from build123d import *

# Parameters (mm, degrees)
SKETCH1_R           = 1.5
BOSS_EXTRUDE1_DEPTH = 2
SKETCH2_R           = 1.5
BOSS_EXTRUDE2_DEPTH = 5
CUT_EXTRUDE1_DEPTH  = 2
SKETCH5_W           = 3
SKETCH5_H           = 1
CUT_EXTRUDE2_DEPTH  = 22


with BuildPart() as part:
    # Sketch1 → Boss-Extrude1 (new body)
    with BuildSketch(Plane.XY):
        Polygon((-8, 3.5), (-6, 5.5), (6, 5.5), (8, 3.5), (8, -3.5), (6, -5.5), (-6, -5.5), (-8, -3.5), align=None)
        with Locations((-2.5, 0)):
            Circle(SKETCH1_R, mode=Mode.SUBTRACT)
        with Locations((2.5, 0)):
            Circle(SKETCH1_R, mode=Mode.SUBTRACT)
    extrude(amount=BOSS_EXTRUDE1_DEPTH)

    # Sketch2 → Boss-Extrude2 (add)
    with BuildSketch(Plane.XY.offset(2)):
        with BuildLine():
            Line((-2.5, 4.5), (2.5, 4.5))
            ThreePointArc((2.5, 4.5), (7, 0), (2.5, -4.5))
            Line((2.5, -4.5), (-2.5, -4.5))
            ThreePointArc((-2.5, -4.5), (-7, 0), (-2.5, 4.5))
        make_face()
        with Locations((-2.5, 0)):
            Circle(SKETCH2_R, mode=Mode.SUBTRACT)
        with Locations((2.5, 0)):
            Circle(SKETCH2_R, mode=Mode.SUBTRACT)
    extrude(amount=BOSS_EXTRUDE2_DEPTH)

    # Sketch4 → Cut-Extrude1 (cut)
    with BuildSketch(Plane.XY.offset(7)):
        with BuildLine():
            Line((-2.5, -2.5), (2.5, -2.5))
            ThreePointArc((2.5, -2.5), (3.618033989, -2.236067977), (4.5, -1.5))
            Line((4.5, -1.5), (7.291771179, -1.5))
            Line((7.291771179, -1.5), (6.980260776, 3.5))
            Line((6.980260776, 3.5), (4.540127242, 3.5))
            Line((4.540127242, 3.5), (-4.895055756, 3.5))
            Line((-4.895055756, 3.5), (-6.610543574, 3.5))
            Line((-6.610543574, 3.5), (-7.482128219, -1.5))
            Line((-7.482128219, -1.5), (-4.5, -1.5))
            ThreePointArc((-4.5, -1.5), (-3.618033989, -2.236067977), (-2.5, -2.5))
        make_face()
    extrude(amount=-CUT_EXTRUDE1_DEPTH, mode=Mode.SUBTRACT)

    # Sketch5 → Cut-Extrude2 (cut)
    with BuildSketch(Plane.ZY.offset(8)):
        with Locations((5.5, 4)):
            Rectangle(SKETCH5_W, SKETCH5_H)
    extrude(amount=-CUT_EXTRUDE2_DEPTH, mode=Mode.SUBTRACT)


solid = part.part
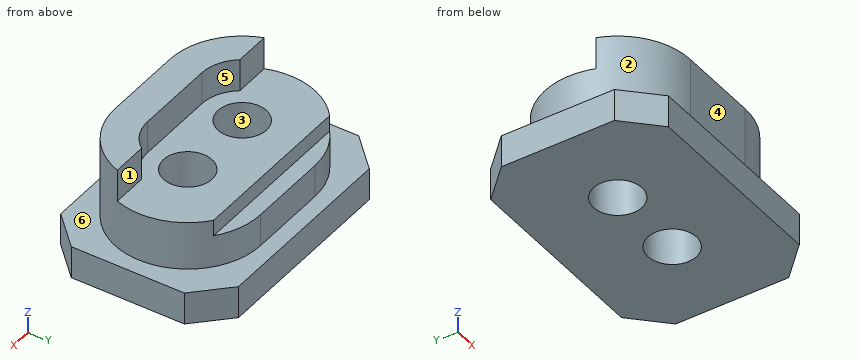
Here's how the part is built. I have some questions about the finished solid (model axes, mm). Face numbers are marked on the shaded views. A direction names the side the tool comes from. Give positions to 0.01 mm unless a question says otherwise; leave off trailing zeros. Loops run counter-clockwise (first coordinate to the right, second up) from the corner with the lowest first, then second, coordinate; pieces in that order, holes last. Notation, with made-up numbers: (16.5, 63.25) -> (44.5, 63.25) arc R12 cw to (44.5, 72.25) -> close; hole circle Ø2 at (-37, 7.5). An arc over 180 degrees is marked (long way). Answer as a JSON object with one key per item and string values. Group by question number.
Item 1: Imagine slicing it at B-B on y = 0. Write out the boundary of the cut face in (x, z).
Item 2: Thinking about a two-plate mould opening in X: for the marked faces 1, 2 and 3, which applies, pulls with the +X half, pulls with the -X half, needs draft (parallel to the pull), parting line crosses it, or undercut?
Item 3: Imagine slicing it at A-A on z = 0.5. Write out the boundary of the cut face in (x, y).
Item 4: On a 3-axis mill with a long thin cutter (end or side, diameter ignored), from which of +Z, -Z, +X, -X, +Y, -Y can I reach the whole of each face in a straight line? I mean the marked faces 4, 5 and 6. Say none if no direction works.
Item 5: Imagine slicing it at D-D on z = 5.25. Write out the boundary of the cut face in (x, y), then the cut area to 3 significant figures.
Item 6: Imagine slicing it at C-C on x = 2. Write out the boundary of the cut face in (y, z).
Item 7: Will these pins go through, and if not, where does the flat tip stop? pin 1 (0.8 mm diameter, centred on x = 0, z = 4.5, fed in from +Y); pin 2 (1.6 mm diameter, centred on x = -6, z = 6, fed in from +Y); pin 3 (0.6 mm diameter, centred on x = -1, z = 3, fed in from +Y); pin 4 (1.8 mm diameter, centred on x = 2.5, y = 0, fed in from +Z).
Item 8: I need wall thicknesses on L1, parallel to X at y = 0, z = 2.65; L2, parallel to X at y = 0, z = 1.35; L3, parallel to Y at x = -2.5, z = 0.5. Which ranges of each line are inside material? Lowest first, please.
Answer list:
{
 "1": {"outline": "(-8, 0) -> (-4, 0) -> (-4, 5) -> (-7, 5) -> (-7, 2) -> (-8, 2) -> close; (-1, 0) -> (1, 0) -> (1, 5) -> (-1, 5) -> close; (4, 0) -> (8, 0) -> (8, 2) -> (7, 2) -> (7, 5) -> (4, 5) -> close"},
 "2": {"face 1": "needs draft", "face 2": "pulls with the -X half", "face 3": "undercut"},
 "3": {"outline": "(-8, -3.5) -> (-6, -5.5) -> (6, -5.5) -> (8, -3.5) -> (8, 3.5) -> (6, 5.5) -> (-6, 5.5) -> (-8, 3.5) -> close; hole circle Ø3 at (-2.5, 0); hole circle Ø3 at (2.5, 0)"},
 "4": {"face 4": "+Z, +X, -X, -Y", "face 5": "+Z, +Y", "face 6": "+Z"},
 "5": {"outline": "(-6.74, -1.5) arc R4.5 ccw to (-2.5, -4.5) -> (2.5, -4.5) arc R4.5 ccw to (6.74, -1.5) -> (4.5, -1.5) arc R2.5 cw to (2.5, -2.5) -> (-2.5, -2.5) arc R2.5 cw to (-4.5, -1.5) -> close", "area": "25.8 mm2"},
 "6": {"outline": "(-5.5, 0) -> (-1.41, 0) -> (-1.41, 5) -> (-2.5, 5) -> (-2.5, 7) -> (-4.5, 7) -> (-4.5, 2) -> (-5.5, 2) -> close; (1.41, 0) -> (5.5, 0) -> (5.5, 2) -> (4.5, 2) -> (4.5, 4) -> (3.5, 4) -> (3.5, 5) -> (1.41, 5) -> close"},
 "7": {"pin 1": "stops at y = 3.5", "pin 2": "stops at y = -1.5", "pin 3": "stops at y = 4.5", "pin 4": "passes through"},
 "8": {"L1": "x = -7 to -4, -1 to 1, 4 to 7", "L2": "x = -8 to -4, -1 to 1, 4 to 8", "L3": "y = -5.5 to -1.5, 1.5 to 5.5"}
}
